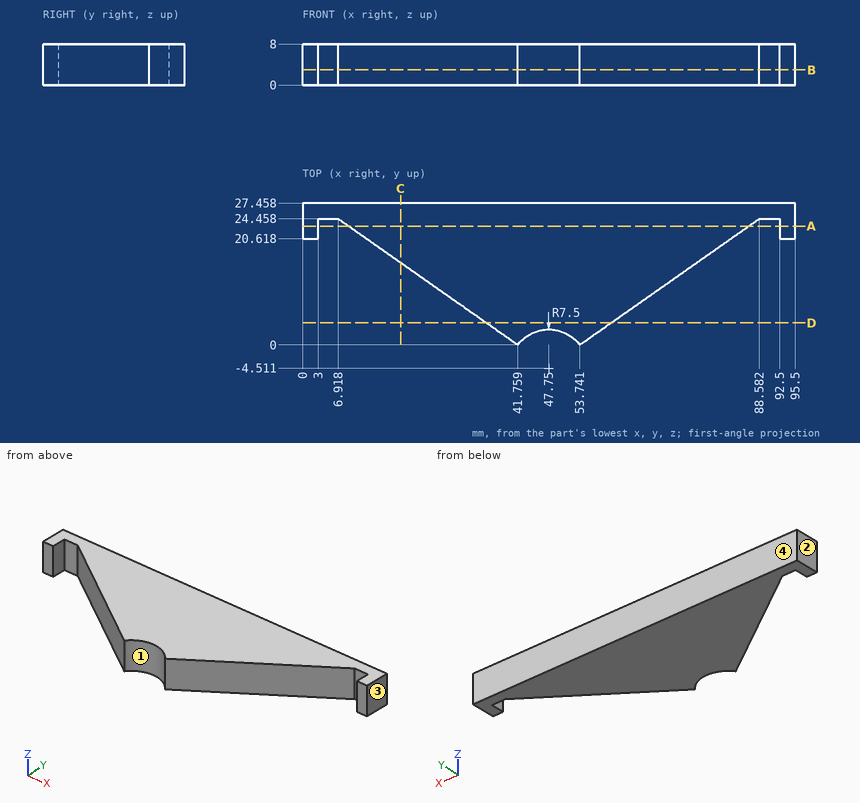
Verification items for this drawing (mm, ordinates from the low corner). Coordinates: 2 decimals unless noted, no trailing zeros. Loops run counter-clockwise (first coordinate to the right, second up) from the corner with the lowest first, then second, coordinate; pieces in that order, holes last. Notation, with made-up numbers: (11, -8) -> (32, -8) arc R8 cw to (32, 7) -> close; hole circle Ø5 at (17, -39). An arc over 180 degrees is marked (long way). Answer in a Markdown table with one row per item. Add a question column.
1. Section check C-C, the plane x = 19. Enter the section's corners in (y, z).
2. Section check B-B, the plane z = 3. Enter the section's corners in (x, y).
3. Section check D-D, the plane y = 4.25. Enter the section's corners in (x, z) (1 decimal), then the cut area to 3 significant figures.
4. Draft check along X on the marked faces 1, 2, 3 and 4. Enter one of: +X half, -X half, draft (parallel to the pull), parting line (faces both ways), or undercut.
5. Section check A-A, the plane y = 23. Enter the section's corners in (x, z) (1 decimal).
6. Material ranges on probe 1 along X at (y, z) = (9.25, 2) (1 decimal); probe 2 along X at (y, z) = (10.5, 3.5); probe 3 along Y at (x, z) = (71.5, 1) (1 decimal), recorded low to high. Write a range as [from, to].
7. Depth check by flat-ended pin: P1, Ø2.5, axis at x = 2, z = 3, coming from the -Y side; P2, Ø3, axis at y = 5.5, z = 2.5, coming from the +X side (1 decimal); P3, Ø1, axis at x = 49, y = 8.5, coming from the -Z side; P4, Ø1.2, axis at x = 4, z = 3, coming from the -Y side. Enter the tip coordinate at first touch or a pass-through.
Derived:
| question | item | result |
|---|---|---|
| 1 | outline | (15.98, 0) -> (27.46, 0) -> (27.46, 8) -> (15.98, 8) -> close |
| 2 | outline | (0, 20.62) -> (3, 20.62) -> (3, 24.46) -> (6.92, 24.46) -> (41.76, 0) arc R7.5 cw to (53.74, 0) -> (88.58, 24.46) -> (92.5, 24.46) -> (92.5, 20.62) -> (95.5, 20.62) -> (95.5, 27.46) -> (0, 27.46) -> close |
| 3 | outline | (35.7, 0) -> (59.8, 0) -> (59.8, 8) -> (35.7, 8) -> close |
| 3 | area | 193 mm² |
| 4 | face 1 | undercut |
| 4 | face 2 | -X half |
| 4 | face 3 | +X half |
| 4 | face 4 | draft |
| 5 | outline | (0, 0) -> (3, 0) -> (3, 8) -> (0, 8) -> close; (9, 0) -> (86.5, 0) -> (86.5, 8) -> (9, 8) -> close; (92.5, 0) -> (95.5, 0) -> (95.5, 8) -> (92.5, 8) -> close |
| 6 | probe 1 | x = [28.6, 66.9] |
| 6 | probe 2 | x = [26.8, 68.7] |
| 6 | probe 3 | y = [12.5, 27.5] |
| 7 | P1 | stops at y = 20.62 |
| 7 | P2 | stops at x = 63.7 |
| 7 | P3 | stops at z = 0 |
| 7 | P4 | stops at y = 24.46 |
